from build123d import *

# Parameters (mm, degrees)
F2_DEPTH = 1.905
F3_DEPTH = 3.81


with BuildPart() as f2:
    # F0 (on Front) → F2 (new body)
    with BuildSketch(Plane.XZ):
        with BuildLine():
            Line((-76.2, 15.875), (-76.2, 0))
            Line((-76.2, 0), (-60.325, 0))
            ThreePointArc((-60.325, 0), (-64.9746798487, 11.2253201513), (-76.2, 15.875))
        make_face()
        with BuildLine():
            Line((-60.325, 0), (-76.2, 0))
            Line((-76.2, 0), (-76.2, -15.875))
            ThreePointArc((-76.2, -15.875), (-64.9746798487, -11.2253201513), (-60.325, 0))
        make_face()
        with BuildLine():
            Line((-76.2, -15.875), (-76.2, 0))
            Line((-76.2, 0), (-76.2, 15.875))
            ThreePointArc((-76.2, 15.875), (-92.075, 0), (-76.2, -15.875))
        make_face()
        with BuildLine():
            ThreePointArc((-76.2, 15.875), (-64.9746798487, 11.2253201513), (-60.325, 0))
            Line((-60.325, 0), (60.325, 0))
            ThreePointArc((60.325, 0), (64.9746798487, 11.2253201513), (76.2, 15.875))
            Line((76.2, 15.875), (-76.2, 15.875))
        make_face()
        with BuildLine():
            Line((60.325, 0), (-60.325, 0))
            ThreePointArc((-60.325, 0), (-64.9746798487, -11.2253201513), (-76.2, -15.875))
            Line((-76.2, -15.875), (76.2, -15.875))
            ThreePointArc((76.2, -15.875), (64.9746798487, -11.2253201513), (60.325, 0))
        make_face()
        with BuildLine():
            ThreePointArc((76.2, 15.875), (64.9746798487, 11.2253201513), (60.325, 0))
            Line((60.325, 0), (76.2, 0))
            Line((76.2, 0), (76.2, 15.875))
        make_face()
        with BuildLine():
            Line((76.2, 0), (60.325, 0))
            ThreePointArc((60.325, 0), (64.9746798487, -11.2253201513), (76.2, -15.875))
            Line((76.2, -15.875), (76.2, 0))
        make_face()
        with BuildLine():
            Line((76.2, 0), (76.2, -15.875))
            ThreePointArc((76.2, -15.875), (87.4253201513, -11.2253201513), (92.075, 0))
            ThreePointArc((92.075, 0), (87.4253201513, 11.2253201513), (76.2, 15.875))
            Line((76.2, 15.875), (76.2, 0))
        make_face()
    extrude(amount=F2_DEPTH)

    # F1 (on Front) → F3 (join)
    with BuildSketch(Plane.XZ):
        with BuildLine():
            ThreePointArc((76.2, -13.97), (62.23, 0), (76.2, 13.97))
            Line((76.2, 13.97), (-76.2, 13.97))
            ThreePointArc((-76.2, 13.97), (-66.3217182668, 9.8782817332), (-62.23, 0))
            ThreePointArc((-62.23, 0), (-66.3217182668, -9.8782817332), (-76.2, -13.97))
            Line((-76.2, -13.97), (76.2, -13.97))
        make_face()
        with BuildLine():
            ThreePointArc((90.17, 0), (86.0782817332, 9.8782817332), (76.2, 13.97))
            Line((76.2, 13.97), (76.2, -13.97))
            ThreePointArc((76.2, -13.97), (86.0782817332, -9.8782817332), (90.17, 0))
        make_face()
        with BuildLine():
            Line((76.2, -13.97), (76.2, 13.97))
            ThreePointArc((76.2, 13.97), (62.23, 0), (76.2, -13.97))
        make_face()
        with BuildLine():
            ThreePointArc((-62.23, 0), (-66.3217182668, 9.8782817332), (-76.2, 13.97))
            Line((-76.2, 13.97), (-76.2, -13.97))
            ThreePointArc((-76.2, -13.97), (-66.3217182668, -9.8782817332), (-62.23, 0))
        make_face()
        with BuildLine():
            Line((-76.2, -13.97), (-76.2, 13.97))
            ThreePointArc((-76.2, 13.97), (-90.17, 0), (-76.2, -13.97))
        make_face()
    extrude(amount=-F3_DEPTH)


solid = f2.part
The model under review builds one solid part; all positions refer to its coordinate system, in mm. A direction names the side the tool comes from. Give positions to 0.01 mm unless a question says otherwise; leave off trailing zeros. Loops run counter-clockwise (first coordinate to the right, second up) from the corner with the lowest first, then second, coordinate; pieces in that order, holes last. Notation, with made-up numbers: (88, 16) -> (117, 16) arc R14 cw to (117, 40) -> close; hole circle Ø5 at (-39.5, 70.25). An arc over 180 degrees is marked (long way). Answer as a JSON object with one key per item and string values. Group by question number.
Q1. Wall thickness on line 1 along Z through (x, y) = (-64, 3.05); line 2 along Y through (x, z) = (82, 14) (3 decimals); line 3 along X through (y, z) = (3.45, 0.5): over which ranges is each line inside the solid? List them lowest first.
Q2. Insertion check: pin 1 (1 mm diameter, centred on y = 2.5, z = -7.5, fed in from -X); pin 2 (1.9 mm diameter, centred on x = -12.5, y = 1.5, fed in from +Z); pin 3 (3 mm diameter, centred on y = 0.5, z = 8, fed in from +X). Each pin has a flat end and moves straight along its axis. Give the tip position at first contact, or say it passes through.
Q3. Take a section at A-A (x = 67). Write out the cut boundary in (y, z) (3 decimals), plus the area to 3 significant figures.
Q4. Tool access review of faces 1 (the flat face through (1, 2, 13.97)), 2 (the flat face through (-1, 2, -13.97)), 3 (the flat face through (-1, -1.905, 0)), 4 (the cylindrical face through (-90.167, 1.878, 0.307)), 5 (the flat face through (-1, 3.81, 0)): name each direction out of +Z, -Z, +X, -X, +Y, -Y from which nothing blocks a thin tool from reaching the whole face with its end or side.
Q5. Take a section at B-B (z = -2). Write out the cut boundary in (x, y) (3 decimals), plus the area to 3 significant figures.
Answer below:
{
 "1": {"line 1": "z = -13.97 to 13.97", "line 2": "y = -1.905 to 0", "line 3": "x = -90.16 to 90.16"},
 "2": {"pin 1": "stops at x = -88.29", "pin 2": "stops at z = 13.97", "pin 3": "stops at x = 90.64"},
 "3": {"outline": "(-1.905, -15.875) -> (0, -15.875) -> (0, -13.97) -> (3.81, -13.97) -> (3.81, 13.97) -> (0, 13.97) -> (0, 15.875) -> (-1.905, 15.875) -> close", "area": "167 mm2"},
 "4": {"face 1": "+Z, +X, -X, +Y", "face 2": "-Z, +X, -X, +Y", "face 3": "+Z, -Z, +X, -X, -Y", "face 4": "-X, +Y", "face 5": "+Z, -Z, +X, -X, +Y"},
 "5": {"outline": "(-91.949, -1.905) -> (91.949, -1.905) -> (91.949, 0) -> (90.026, 0) -> (90.026, 3.81) -> (-90.026, 3.81) -> (-90.026, 0) -> (-91.949, 0) -> close", "area": "1,040 mm2"}
}
